Read the model definition and answer for the solid it produces. Units are mm, in the model's axes. Coordinates: 2 decimals unless noted, no trailing zeros. Order: outer loops, then holes, each group sorted by start corner. A loop starts at its lowest first (then second) coordinate and runs counter-clockwise, first axis right, second up. Notation, with made-up numbers: (-29, 42) -> (15, 42) arc R19 cw to (15, 58) -> close; hole circle Ø6 at (25, 56.5). An arc over 180 degrees is marked (long way). Answer in a Markdown table with one row per item.
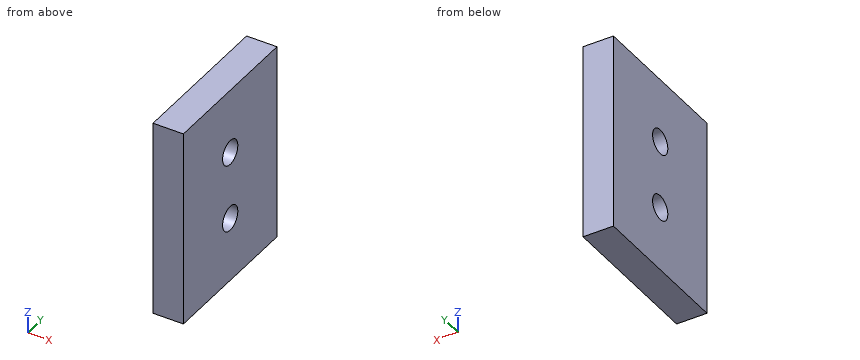
Autodesk Inventor part; units mm, degrees
ref_plane "Startebene" through (0, 0, 0) normal (0, 0, 1) x (1, 0, 0)
ref_plane "Endebene" through (0, 0, 52) normal (0, 0, 1) x (1, 0, 0)
ref_plane "YZ Plane" through (0, 0, 0) normal (1, 0, 0) x (0, 1, 0)
ref_plane "Startebene" through (0, 0, 0) normal (0, 0, 1) x (1, 0, 0)
ref_plane "Endebene" through (0, 0, 52) normal (0, 0, 1) x (1, 0, 0)
sketch "Skizze" plane through (0, 0, 0) normal (0, 0, 1) x (1, 0, 0)
  line L0 (4, -20) -> (-4, -20)
  line L1 (-4, -20) -> (-4, 20)
  line L2 (-4, 20) -> (4, 20)
  line L3 (4, 20) -> (4, -20)
  line L4 (-6, 0) -> (8, 0) construction
  line L5 (0, -30) -> (0, 40) construction
  line L6 (0, 54) -> (0, -44) construction
  line L7 (-9.2, 0) -> (13.2, 0) construction
  dimension "d0" = 40
  dimension "d1" = 8
  dimension "d4" = 4
  dimension "d5" = 20
extrude "Körper" add sketch "Skizze" along normal up to surface (52 mm away) from surface at 0
sketch "Sketch3" plane through (0, 0, 0) normal (0, 0, 1) x (1, 0, 0)
  line L0 (0, 0) -> (10, 0)
ref_plane "Work Plane3" through (0, 0, 0) normal (0, -1, 0) x (1, 0, 0)
sketch "Sketch4" plane through (0, 0, 0) normal (0, -1, 0) x (1, 0, 0)
  line L0 (-2, 0) -> (12, 0)
  line L1 (-2, 52) -> (12, 52)
  dimension "d9" = 52
sketch "Skizze5" plane through (4, -20, 52) normal (1, 0, 0) x (0, 0, -1)
  line L0 (0, 40) -> (0, 0)
  line L1 (52, 0) -> (0, 0)
  line L2 (52, 40) -> (52, 0)
  point P0 (52, 20)
  point P1 (17, 20)
  point P2 (35, 20)
  dimension "d10" = 20
  dimension "d11" = 20
  dimension "d12" = 17
  dimension "d13" = 17
hole "Bohrung1" at (4, 0, 35) at (4, 0, 17) direction (-1, 0, 0) diameter 6.5 depth 35 tip angle 118
equation "\"d0\" = G_W"
equation "\"d1\" = G_H"
equation "\"d4\" = 0.5 * d1"
equation "\"d5\" = 0.5 * d0"
equation "\"d2\" = G_L"
equation "\"G_W\" = 40"
equation "\"G_H\" = 8"
equation "\"G_L\" = d9"
equation "\"G_OFFSET_START\" = 0"
equation "\"G_OFFSET_END\" = 0"
equation "\"d7\" = G_OFFSET_END + B_L"
equation "\"B_L\" = 52"
properties part number "EN 10058 - 40 x 6 - 46" material "Stahl, weich"
Q1. The part is cut by section B-B (z = 17). Write down the section's boundary in (x, y), then the cut area to 3 significant figures.
Outcome:
| item | result |
|---|---|
| outline | (-4, -20) -> (4, -20) -> (4, -3.25) -> (-4, -3.25) -> close; (-4, 3.25) -> (4, 3.25) -> (4, 20) -> (-4, 20) -> close |
| area | 268 mm² |
Q2. The part is cut by section A-A (y = 0). Write down the section's boundary in (x, z), then the cut area to 3 significant figures.
Outcome:
| item | result |
|---|---|
| outline | (-4, 0) -> (4, 0) -> (4, 13.75) -> (-4, 13.75) -> close; (-4, 20.25) -> (4, 20.25) -> (4, 31.75) -> (-4, 31.75) -> close; (-4, 38.25) -> (4, 38.25) -> (4, 52) -> (-4, 52) -> close |
| area | 312 mm² |
Q3. The part is cut by section C-C (x = -2.5). Write down the section's boundary in (y, z), then the cut area to 3 significant figures.
Outcome:
| item | result |
|---|---|
| outline | (-20, 0) -> (20, 0) -> (20, 52) -> (-20, 52) -> close; hole circle Ø6.5 at (0, 17); hole circle Ø6.5 at (0, 35) |
| area | 2,010 mm² |
Q4. Given pin 1 (4 mm diameter, centred on y = 0, z = 17, fed in from +X), flat-ended and moving along its own axis, determine where the tip first touches the part or whether it passes through.
Outcome:
| item | result |
|---|---|
| pin 1 | through |
Q5. Consider line 1 (Z direction, x = 2.25, y = 0); line 2 (Y direction, x = 0.5, z = 17); line 3 (Y direction, x = -3.5, z = 36). Determine where each line is inside the solid, lowest interval first.
Outcome:
| item | result |
|---|---|
| line 1 | 0 to 13.75, 20.25 to 31.75, 38.25 to 52 |
| line 2 | -20 to -3.25, 3.25 to 20 |
| line 3 | -20 to -3.09, 3.09 to 20 |
